```python
from build123d import *

# Parameters (mm, degrees)
CUT_EXTRUDE3_DEPTH         = 1.9746
DRAFT1_ANGLE               = 20
RECESSI_CUT_EXTRUDE5_DEPTH = 1.9746


with BuildPart() as part:
    # Sketch1 → base-Revolve (revolve)
    with BuildSketch(Plane.XY, mode=Mode.PRIVATE) as base_revolve_sk:
        with BuildLine():
            Line((0, 0), (0, 2.2606))
            ThreePointArc((0, 2.2606), (0.342216437, 3.086783563), (1.1684, 3.429))
            Line((1.1684, 3.429), (2, 3.429))
            Line((2, 3.429), (2, 1.5))
            Line((2, 1.5), (27, 1.5))
            Line((27, 1.5), (27, 0))
            Line((27, 0), (0, 0))
        make_face()
    revolve(base_revolve_sk.sketch.rotate(Axis((0, 0, 0), (1, 0, 0)), 90), axis=Axis((0, 0, 0), (1, 0, 0)))

    # Sketch4 → Cut-Extrude3 (cut)
    with BuildSketch(Plane(origin=(0, 0, 0), x_dir=(0, 0, -1), z_dir=(1, 0, 0))):
        Polygon((0.3556, 2.032), (-0.3556, 2.032), (-0.3556, 0.3556), (-2.032, 0.3556), (-2.032, -0.3556), (-0.3556, -0.3556), (-0.3556, -2.032), (0.3556, -2.032), (0.3556, -0.3556), (2.032, -0.3556), (2.032, 0.3556), (0.3556, 0.3556), align=None)
    extrude(amount=CUT_EXTRUDE3_DEPTH, mode=Mode.SUBTRACT)

    # Draft1
    draft1_faces = [part.faces().sort_by_distance(p)[0] for p in [
        (0.9873, 0, -2.032),
        (0.9873, -2.032, 0),
        (0.9873, 0, 2.032),
        (0.9873, 2.032, 0),
    ]]
    draft(draft1_faces, Plane(origin=(0, 0, 0), x_dir=(0, 0, -1), z_dir=(-1, 0, 0)), DRAFT1_ANGLE)

    # Sketch5 → recessI_Cut-Extrude5 (cut)
    with BuildSketch(Plane.ZY):
        Polygon((0.3556, 0.762), (0.762, 0.3556), (0.3556, 0.3556), align=None)
        Polygon((-0.3556, 0.3556), (-0.762, 0.3556), (-0.3556, 0.762), align=None)
        Polygon((-0.3556, -0.762), (-0.762, -0.3556), (-0.3556, -0.3556), align=None)
        Polygon((0.3556, -0.3556), (0.762, -0.3556), (0.3556, -0.762), align=None)
    extrude(amount=-RECESSI_CUT_EXTRUDE5_DEPTH, mode=Mode.SUBTRACT)

    # Sketch14 → point_Cut-Revolve3 (revolve, cut)
    with BuildSketch(Plane.XY, mode=Mode.PRIVATE) as point_cut_revolve3_sk:
        Polygon((27, 0), (23.783239619, 1.5), (27.184454292, 1.5), (27.184454292, 0), align=None)
    revolve(point_cut_revolve3_sk.sketch.rotate(Axis((0, 0, 0), (1, 0, 0)), 90), axis=Axis((0, 0, 0), (1, 0, 0)), mode=Mode.SUBTRACT)


solid = part.part
```
Input: part model. Units: mm. Frame: model coordinates. A direction names the side the tool comes from. Coordinates: 2 decimals unless noted, no trailing zeros. Loops run counter-clockwise (first coordinate to the right, second up) from the corner with the lowest first, then second, coordinate; pieces in that order, holes last.
Q1. Mould query, pull axis Z, two halves, no side actions, for faces 1 (the flat face through (1, 1, 0.356)), 2 (the conical face through (25.727, 0.527, 0.274)), 3 (the flat face through (0, -1, -1)), 4 (the flat face through (1, 0.356, -1)). Classes: +Z half, -Z half, draft (parallel to the pull), parting line (faces both ways), or undercut.
Results are:
face 1: undercut
face 2: parting line
face 3: draft
face 4: undercut
Q2. Line query: line 1 along X through (y, z) = (-1.5, 0.5); line 2 along Y through (x, z) = (12.5, 0); line 3 along X through (y, z) = (-1, -3). Output: solid intervals per line, ascending.
Results are:
line 1: x = 0 to 2
line 2: y = -1.5 to 1.5
line 3: x = 0.43 to 2
Q3. Set-up query: faces 5 (the cylindrical face through (13.04, -0.45, 1.43)), 6 (the flat face through (1, 1, -0.356)), 7 (the cylindrical face through (1.59, 3.35, -0.74)). Return all of +Z, -Z, +X, -X, +Y, -Y with unobstructed straight access to the full face (end or side cutting, diameter ignored); none if empty.
Results are:
face 5: +X
face 6: -X
face 7: +X, -X
Q4. Section A-A, the plane x = 15.5. Return the cut outline in (y, z).
Results are:
outline: circle Ø3 at (0, 0)
Q5. Contact query for flat-ended pins moving along their axis: pin 1 (0.6 mm diameter, centred on x = 1, y = -1.5, fed in from -Z); pin 2 (1.5 mm diameter, centred on x = 6.5, z = 1, fed in from +Y); pin 3 (1 mm diameter, centred on x = 1, y = -1, fed in from +Z). Output: stop coordinate, or through.
Results are:
pin 1: stops at z = -3.2
pin 2: stops at y = 1.48
pin 3: stops at z = 3.39
